Autodesk Inventor part; units mm, degrees
ref_plane "YZ Plane" through (0, 0, 0) normal (1, 0, 0) x (0, 1, 0)
ref_plane "XZ Plane" through (0, 0, 0) normal (0, 1, 0) x (-1, 0, 0)
ref_plane "XY Plane" through (0, 0, 0) normal (0, 0, 1) x (1, 0, 0)
sketch "Sketch1" plane through (0, 0, 0) normal (0, 0, 1) x (1, 0, 0)
  arc A0 (368.3, 25.4) -> (578.4957, 191.999) centre (368.3, 241.3) ccw
  arc A1 (368.3, 0) -> (603.2246, 186.1989) centre (368.3, 241.3) ccw
  line L0 (368.3, 25.4) -> (0, 25.4)
  line L1 (0, 25.4) -> (0, 0)
  line L2 (0, 0) -> (368.3, 0)
  line L3 (578.4957, 191.999) -> (603.2246, 186.1989)
  line L4 (368.3, 25.4) -> (368.3, 241.3) construction
  line L5 (368.3, 241.3) -> (578.4957, 191.999) construction
  dimension "d5" = 25.4
  dimension "d6" = 215.9
  dimension "d7" = 368.3
  dimension "d8" = 76.8
extrude "Extrusion1" add sketch "Sketch1" along normal blind 25.4
shell "Shell1" thickness 1.5875 removed faces 2 at (0, 8.4667, 8.4667) at (586.7387, 190.0657, 16.9333)
properties part number "Frame_RearBallGuide"
Build history of the part. All positions in model axes, mm. A direction names the side the tool comes from. Round coordinates to 2 decimals unless told otherwise and drop trailing zeros. Write each loop counter-clockwise with the first axis right and the second up, starting at its lowest first coordinate (ties: lowest second). Pieces come first, ordered by that corner, then holes. Notation, with made-up numbers: M 41.25,-9 L 100.25,-9 A16 ccw 100.25,2 Z; hole C 2,-10.5 d1. An arc over 180 degrees is marked long. Answer as a JSON object with one key per item and string values. Group by question number.
(1) Cut at A-A (z = 13.25). Give the cut face in (x, y).
(2) Cut at B-B (y = 104.5). Give the cut face in (x, z), and give its area (3 significant figures).
(3) Mould opens along X. For faces 1 (the cylindrical face through (504.985, 72.131, 12.544)), 2 (the flat face through (182, 0, 13)), 3 (the cylindrical face through (503.99, 73.37, 12.52)) say: pulls with the +X half, pulls with the -X half, needs draft (parallel to the pull), parting line crosses it, or undercut.
(4) Cut at D-D (y = 14). Give the cut face in (x, z), and give its area (3 significant figures).
(5) Which spindle directions (+Z, -Z, +X, -X, +Y, -Y) get a long thin tool onto all of the face, cutting with end or side? Do faces 4 (the flat face through (182, 1.588, 13)), 5 (the cylindrical face through (518.95, 54.84, 12.54)), 6 (the flat face through (187, 25.4, 13)), 7 (the flat face through (323, 25, 25.4)). Say none if no direction does.
(6) Flat gauge pins, fed straight in: pin 1 (4 mm diameter, centred on x = 125.5, z = 11.5, fed in from -Y); pin 2 (6 mm diameter, centred on y = 137.5, z = 2.5, fed in from +X); pin 3 (11 mm diameter, centred on x = 145, z = 12, fed in from +Y); pin 4 (4 mm diameter, centred on y = 84, z = 18.5, fed in from -X). Where does each tip first touch, or does it go through?
(7) Drill centre lines: L1, parallel to Y at x = 54.5, z = 7; L2, parallel to X at y = 68, z = 8.75. Where is each one in solid material? Low to high.
(8) Cut at C-C (x = 63.5). Give the cut face in (y, z), and give its area (3 significant figures).
Responses:
{
 "1": {"outline": "M 0,0 L 368.3,0 A241.3 ccw 603.22,186.2 L 601.68,186.56 A239.71 cw 368.3,1.59 L 0,1.59 Z; M 0,23.81 L 368.3,23.81 A217.49 ccw 580.04,191.64 L 578.5,192 A215.9 cw 368.3,25.4 L 0,25.4 Z"},
 "2": {"outline": "M 535.33,0 L 567.07,0 L 567.07,25.4 L 535.33,25.4 Z; hole M 537.38,1.59 L 565.14,1.59 L 565.14,23.81 L 537.38,23.81 Z", "area": "189 mm2"},
 "3": {"face 1": "undercut", "face 2": "needs draft", "face 3": "pulls with the -X half"},
 "4": {"outline": "M 0,0 L 449.3,0 L 449.3,25.4 L 0,25.4 L 0,23.81 L 444.44,23.81 L 444.44,1.59 L 0,1.59 Z", "area": "1,530 mm2"},
 "5": {"face 4": "-X", "face 5": "none", "face 6": "+Z, -Z, -X, +Y", "face 7": "+Z, +X, -X, +Y, -Y"},
 "6": {"pin 1": "stops at y = 0", "pin 2": "stops at x = 587.54", "pin 3": "stops at y = 25.4", "pin 4": "stops at x = 514.03"},
 "7": {"L1": "y = 0 to 1.59, 23.81 to 25.4", "L2": "x = 497.06 to 499.71, 533.92 to 536.21"},
 "8": {"outline": "M 0,0 L 25.4,0 L 25.4,25.4 L 0,25.4 Z; hole M 1.59,1.59 L 23.81,1.59 L 23.81,23.81 L 1.59,23.81 Z", "area": "151 mm2"}
}
